Could you check a few things on this model? Use its own coordinates, in mm. A direction names the side the tool comes from. Give positions to 0.01 mm unless a question says otherwise; leave off trailing zeros. Write each loop counter-clockwise with the first axis right and the second up, starting at its lowest first coordinate (ties: lowest second). Pieces come first, ordered by that corner, then holes. Notation, with made-up numbers: (83.25, 35) - (116.25, 35) arc R11 ccw to (116.25, 55) - close; hole circle Ø3 at (-39, 56.25). An arc over 180 degrees is marked (long way). Write item = value, one per line.
from build123d import *

# Parameters (mm, degrees)
F0_W     = 42
F0_H     = 43
F0_R     = 0.75
F0_W_2   = 30.5
F0_H_2   = 34.5
F1_DEPTH = 2
F2_W     = 5.75
F2_H     = 10
F2_R     = 0.75
F2_W_2   = 10
F2_H_2   = 5.5
F3_DEPTH = 2
F4_R     = 8.4
F5_DEPTH = 3
F6_R     = 1.99999
F7_R     = 1


# Not quite as in the source:
# - a fillet or chamfer is up to 0.001 mm smaller than in the source, because OpenCascade refuses the exact size


with BuildPart() as f1:
    # F0 (on Top) → F1 (new body)
    with BuildSketch(Plane.XY):
        with Locations((0, -18.5)):
            Rectangle(F0_W, F0_H)
        with Locations((0, -37)):
            Circle(F0_R, mode=Mode.SUBTRACT)
        with Locations((-18, -5)):
            Circle(F0_R, mode=Mode.SUBTRACT)
        with Locations((0, -17.25)):
            Rectangle(F0_W_2, F0_H_2, mode=Mode.SUBTRACT)
        with Locations((18, -5)):
            Circle(F0_R, mode=Mode.SUBTRACT)
    extrude(amount=F1_DEPTH)

    # F2 (on face) → F3 (join)
    with BuildSketch(Plane.XY.offset(2)):
        with Locations((-18.125, -5)):
            Rectangle(F2_W, F2_H)
        with Locations((-18, -5)):
            Circle(F2_R, mode=Mode.SUBTRACT)
        with Locations((18.125, -5)):
            Rectangle(F2_W, F2_H)
        with Locations((18, -5)):
            Circle(F2_R, mode=Mode.SUBTRACT)
        with Locations((0, -37.25)):
            Rectangle(F2_W_2, F2_H_2)
        with Locations((0, -37)):
            Circle(F2_R, mode=Mode.SUBTRACT)
    extrude(amount=F3_DEPTH)

    # F4 (on face) → F5 (cut, through all)
    with BuildSketch(Plane(origin=(0, 3, 0), x_dir=(-1, 0, 0), z_dir=(0, 1, 0))):
        with Locations((-8.75, 9)):
            Circle(F4_R)
        with Locations((8.75, 9)):
            Circle(F4_R)
    extrude(amount=-F5_DEPTH, mode=Mode.SUBTRACT)

    # F6 (radius 2 in the source; OpenCascade refuses exactly that, so slightly less here)
    f6_edges = [f1.edges().sort_by_distance(p)[0] for p in [
        (5, -37.25, 2),
        (18.125, -10, 2),
        (-18.125, -10, 2),
        (-5, -37.25, 2),
        (18.125, 0, 2),
        (-18.125, 0, 2),
    ]]
    fillet(f6_edges, radius=F6_R)

    # F7
    f7_edges = [f1.edges().sort_by_distance(p)[0] for p in [
        (-21, -40, 1),
        (-21, 3, 1),
        (21, -40, 1),
        (21, 3, 1),
    ]]
    fillet(f7_edges, radius=F7_R)


solid = f1.part
1. Thinking about a two-plate mould opening in Y: for faces 4 (the face through (-15.25, -12.4, 1.5)), 5 (the face through (0.403, -36.368, 1.972)), 6 (the face through (-18.08, 0.6, 2.57)), 7 (the face through (21, -14.2, 1.5)), which applies, pulls with the +Y half, pulls with the -Y half, needs draft (parallel to the pull), parting line crosses it, or undercut?
Filled sheet:
face_4 = undercut
face_5 = undercut
face_6 = pulls with the +Y half
face_7 = needs draft
2. Which directions (+Z, -Z, +X, -X, +Y, -Y) give clear straight access to the entire face, cutting with the end or side of a thin tool? Please do faces 1 (the face through (0, -40, 2)), 2 (the face through (0, -34.5, 2)), 3 (the face through (-16.4, 2.2, 2)).
Filled sheet:
face_1 = +Z, -Z, +X, -X, -Y
face_2 = +Z, -Z
face_3 = +Z, +Y
3. I need wall thicknesses on line 1 (Y direction, x = 0, z = 0.7); line 2 (Y direction, x = -14.5, z = 1.05); line 3 (Y direction, x = 0, z = 2.75). Which ranges of each line are inside material? Lowest first, please.
Filled sheet:
line_1 = -40 to -37.75, -36.25 to -34.5, 0 to 3
line_2 = -40 to -34.5, 0 to 3
line_3 = -40 to -37.75, -36.25 to -34.5
4. For pin 1 (7 mm diameter, centred on x = -11.5, y = -24.5, fed in from +Z); pin 2 (4 mm diameter, centred on x = 14.5, y = -26.5, fed in from +Z); pin 3 (1 mm diameter, centred on x = 7.5, z = 1.5, fed in from +Y); pin 4 (1.5 mm diameter, centred on x = -17.5, y = 2, fed in from +Z), each with a flat end and sliding along its axis, tell me the tip position at first contact or that it passes through.
Filled sheet:
pin_1 = through
pin_2 = 2
pin_3 = -34.5
pin_4 = 2.15
5. If we section it at B-B, the plane z = 2.6: Please give me the cut outline in (x, y), and give its area (3 significant figures).
Filled sheet:
outline = (-21, -10.57) - (-15.25, -10.57) - (-15.25, 0.57) - (-21, 0.57) - close; (-5.57, -40) - (5.57, -40) - (5.57, -34.5) - (-5.57, -34.5) - close; (15.25, -10.57) - (21, -10.57) - (21, 0.57) - (15.25, 0.57) - close; hole circle Ø1.5 at (-18, -5); hole circle Ø1.5 at (0, -37); hole circle Ø1.5 at (18, -5)
area = 184 mm2
6. If we section it at A-A, the plane y = -27: Please give me the cut outline in (x, z).
Filled sheet:
outline = (-21, 0) - (-15.25, 0) - (-15.25, 2) - (-21, 2) - close; (15.25, 0) - (21, 0) - (21, 2) - (15.25, 2) - close
7. If we section it at D-D, the plane y = -5: Please give me the cut outline in (x, z), and give its area (3 significant figures).
Filled sheet:
outline = (-21, 0) - (-18.75, 0) - (-18.75, 4) - (-21, 4) - close; (-17.25, 0) - (-15.25, 0) - (-15.25, 4) - (-17.25, 4) - close; (15.25, 0) - (17.25, 0) - (17.25, 4) - (15.25, 4) - close; (18.75, 0) - (21, 0) - (21, 4) - (18.75, 4) - close
area = 34.0 mm2
